The listing builds one solid part. Answer for the finished solid, in the listing's coordinates (mm). A direction names the side the tool comes from. Round coordinates to 2 decimals unless told otherwise and drop trailing zeros. Loops run counter-clockwise (first coordinate to the right, second up) from the corner with the lowest first, then second, coordinate; pieces in that order, holes last. Notation, with made-up numbers: (12, -11.75) - (42, -11.75) arc R17 cw to (42, 0.25) - close; hole circle Ø1 at (-4.5, -34). An arc over 180 degrees is marked (long way). Write item = value, one per line. Start each with the question number.
1) A tool of negligible diameter and unlimited length cuts with its end or side. For faces 1 (the flat face through (3, 1, -6.35)), 2 (the flat face through (8.255, -2, -3)), 3 (the flat face through (4, 0, 0)), 4 (the cylindrical face through (-7.531, -1.628, 5.586)), from which of +Z, -Z, +X, -X, +Y, -Y can it reach the whole face along a straight path? Write none if from no direction.
2) Straight lines are drawn through the part: line 1 along Z through (x, y) = (5, 2); line 2 along Z through (x, y) = (13, -1.25). For each, find the intervals that lie inside material, in ascending order.
3) For a pull along X with two mould halves and no side action, classify faces 5 (the flat face through (-8.255, 2, -2)), 6 (the cylindrical face through (3.463, 1.628, -0.455)), 7 (the flat face through (8.255, 2, 1)) as released by +X, released by -X, zero draft, split by the parting line, or undercut.
4) Section A-A, the plane x = 0 is taken. Determine the outline of the cut face in (y, z).
5) Given pin 1 Ø3.5 at (y, z) = (1, 0.5) entering from +X (3 decimals); pin 2 Ø5 at (x, z) = (3.5, 2.5) entering from -Y; pin 3 Ø3 at (x, y) = (47.5, -2) entering from +Z, each flat-ended and moving along its own axis, determine where each tip first touches the part or whether it passes through.
from build123d import *

# Parameters (mm, degrees)
SKETCH1_R           = 3.4925
BOSS_EXTRUDE3_DEPTH = 3.302
BOSS_EXTRUDE4_DEPTH = 3.302
BOSS_EXTRUDE5_DEPTH = 3.302
CUT_EXTRUDE1_REACH  = 8.35


with BuildPart() as part:
    # Sketch1 → Boss-Extrude3 (new body)
    with BuildSketch(Plane(origin=(0, 0, 0), x_dir=(1, 0, 0), z_dir=(0, 1, 0))):
        with BuildLine():
            ThreePointArc((-10.47160211, -0.846666667), (-11.327855674, -0.22130784), (-12.364806331, 0))
            Line((-12.364806331, 0), (-33.02, 0))
            add(Edge.make_bspline(
                [(-33.02, 0), (-27.473096433, -6.223159861), (-8.255, -6.35)],
                knots=[0, 0, 0, 1, 1, 1], degree=2))
            Line((-8.255, -6.35), (-8.255, -3.81))
            Line((-8.255, -3.81), (-8.255, 0))
            ThreePointArc((-8.255, 0), (-9.071835946, -1.186398896), (-10.47160211, -0.846666667))
        make_face()
        with BuildLine():
            ThreePointArc((5.715, 6.35), (7.511051224, 5.606051224), (8.255, 3.81))
            Line((8.255, 3.81), (8.255, -3.81))
            ThreePointArc((8.255, -3.81), (7.511051224, -5.606051224), (5.715, -6.35))
            Line((5.715, -6.35), (-5.715, -6.35))
            ThreePointArc((-5.715, -6.35), (-7.511051224, -5.606051224), (-8.255, -3.81))
            Line((-8.255, -3.81), (-8.255, 3.81))
            ThreePointArc((-8.255, 3.81), (-7.511051224, 5.606051224), (-5.715, 6.35))
            Line((-5.715, 6.35), (5.715, 6.35))
        make_face()
        with Locations(Location((0, 0, 0), (0, 0, 270))):  # turned: the seam where the file's is
            Circle(SKETCH1_R, mode=Mode.SUBTRACT)
        with BuildLine():
            ThreePointArc((-8.255, -3.81), (-7.511051224, -5.606051224), (-5.715, -6.35))
            Line((-5.715, -6.35), (-8.255, -6.35))
            Line((-8.255, -6.35), (-8.255, -3.81))
        make_face()
        with BuildLine():
            Line((8.255, 3.527942587), (8.255, 1.524))
            add(Edge.make_bspline(
                [(8.255, 1.524), (26.922144182, 2.150849617), (62.646246262, 22.822886738), (91.44, 13.97)],
                knots=[0, 0, 0, 0, 1, 1, 1, 1], degree=3))
            add(Edge.make_bspline(
                [(91.44, 13.97), (66.350363848, 33.352051218), (36.841337127, 7.764653999), (8.255, 6.35)],
                knots=[0, 0, 0, 0, 1, 1, 1, 1], degree=3))
            Line((8.255, 6.35), (8.255, 3.81))
            Line((8.255, 3.81), (8.255, 3.527942587))
        make_face()
        with BuildLine():
            Line((8.255, 6.35), (5.715, 6.35))
            ThreePointArc((5.715, 6.35), (7.511051224, 5.606051224), (8.255, 3.81))
            Line((8.255, 3.81), (8.255, 6.35))
        make_face()
    extrude(amount=BOSS_EXTRUDE3_DEPTH)

    # Sketch1_8 → Boss-Extrude4 (add)
    with BuildSketch(Plane(origin=(0, 0, 0), x_dir=(1, 0, 0), z_dir=(0, 1, 0))):
        with BuildLine():
            Line((8.255, 3.527942587), (8.255, 1.524))
            add(Edge.make_bspline(
                [(8.255, 1.524), (26.922144182, 2.150849617), (62.646246262, 22.822886738), (91.44, 13.97)],
                knots=[0, 0, 0, 0, 1, 1, 1, 1], degree=3))
            add(Edge.make_bspline(
                [(91.44, 13.97), (66.350363848, 33.352051218), (36.841337127, 7.764653999), (8.255, 6.35)],
                knots=[0, 0, 0, 0, 1, 1, 1, 1], degree=3))
            Line((8.255, 6.35), (8.255, 3.81))
            Line((8.255, 3.81), (8.255, 3.527942587))
        make_face()
        with BuildLine():
            Line((8.255, 6.35), (5.715, 6.35))
            ThreePointArc((5.715, 6.35), (7.511051224, 5.606051224), (8.255, 3.81))
            Line((8.255, 3.81), (8.255, 6.35))
        make_face()
    extrude(amount=-BOSS_EXTRUDE4_DEPTH)

    # Sketch1_9 → Boss-Extrude5 (add)
    with BuildSketch(Plane(origin=(0, 0, 0), x_dir=(1, 0, 0), z_dir=(0, 1, 0))):
        with BuildLine():
            ThreePointArc((-10.47160211, -0.846666667), (-11.327855674, -0.22130784), (-12.364806331, 0))
            Line((-12.364806331, 0), (-33.02, 0))
            add(Edge.make_bspline(
                [(-33.02, 0), (-27.473096433, -6.223159861), (-8.255, -6.35)],
                knots=[0, 0, 0, 1, 1, 1], degree=2))
            Line((-8.255, -6.35), (-8.255, -3.81))
            Line((-8.255, -3.81), (-8.255, 0))
            ThreePointArc((-8.255, 0), (-9.071835946, -1.186398896), (-10.47160211, -0.846666667))
        make_face()
        with BuildLine():
            ThreePointArc((-8.255, -3.81), (-7.511051224, -5.606051224), (-5.715, -6.35))
            Line((-5.715, -6.35), (-8.255, -6.35))
            Line((-8.255, -6.35), (-8.255, -3.81))
        make_face()
    extrude(amount=-BOSS_EXTRUDE5_DEPTH)

    # Sketch2 → Cut-Extrude1 (cut, up to next)
    with BuildSketch(Plane.XY, mode=Mode.PRIVATE) as cut_extrude1_sk1:
        with BuildLine():
            Line((-33.02, 3.302), (-33.02, -3.053994927))
            add(Edge.make_bspline(
                [(-33.02, -3.053994927), (-28.519594092, 1.640722514), (-22.101826858, 3.211473856), (-13.921878912, 3.302)],
                knots=[0, 0, 0, 0, 0.941080878, 0.941080878, 0.941080878, 0.941080878], degree=3))
            Line((-13.921878912, 3.302), (-33.02, 3.302))
        make_face()
    cut_extrude1_tool1 = extrude(cut_extrude1_sk1.sketch, amount=CUT_EXTRUDE1_REACH, mode=Mode.PRIVATE) & part.part
    add(cut_extrude1_tool1.solids().sort_by_distance((-28.707051, 1.545014, 0))[0], mode=Mode.SUBTRACT)
    # Sketch2 → Cut-Extrude1 (cut, up to next)
    with BuildSketch(Plane.XY, mode=Mode.PRIVATE) as cut_extrude1_sk2:
        with BuildLine():
            Line((-12.364806331, -3.302), (-33.02, -3.302))
            add(Edge.make_bspline(
                [(-12.364806331, -3.302), (-18.804874471, -1.031483357), (-26.812471442, -0.753963495), (-33.02, -3.302)],
                knots=[0, 0, 0, 0, 1, 1, 1, 1], degree=3))
        make_face()
    cut_extrude1_tool2 = extrude(cut_extrude1_sk2.sketch, amount=CUT_EXTRUDE1_REACH, mode=Mode.PRIVATE) & part.part
    add(cut_extrude1_tool2.solids().sort_by_distance((-22.84596, -2.573969, 0))[0], mode=Mode.SUBTRACT)


solid = part.part
Geometry check:
q1.face_1 = -Z, -X, +Y, -Y
q1.face_2 = +Z, -X, -Y
q1.face_3 = -Y
q1.face_4 = -Z, +X, -Y
q2.line_1 = -6.35 to 6.35
q2.line_2 = -6.79 to -2.03
q3.face_5 = released by -X
q3.face_6 = undercut
q3.face_7 = released by +X
q4.outline = (0, -6.35) - (3.3, -6.35) - (3.3, -3.49) - (0, -3.49) - close; (0, 3.49) - (3.3, 3.49) - (3.3, 6.35) - (0, 6.35) - close
q5.pin_1 = 8.255
q5.pin_2 = 0
q5.pin_3 = -11.29
